For this review, take the finished solid that the model builds, in its own axes (mm). A direction names the side the tool comes from. Give positions to 0.01 mm unless a question says otherwise; leave off trailing zeros. Order: outer loops, then holes, each group sorted by start corner. A loop starts at its lowest first (then second) coordinate and runs counter-clockwise, first axis right, second up. Notation, with made-up numbers: (-6, -12) -> (13, -12) arc R20 ccw to (13, 9) -> close; hole circle Ø1 at (-2, -5.5). An arc over 180 degrees is marked (long way). Return JSON: item names as keys, results as strings. Group by question number.
1) Add section C-C (x = 0.7). Give the boundary of the cut face in (y, z).
2) Add section A-A (z = -6.5). Give the boundary of the cut face in (x, y), then the cut area to 3 significant figures.
3) For faces 4 (the face through (0.493, -11.716, 4.264)), 5 (the face through (0.49, 11.19, 0.42)), list the 3-axis set-ups (+Z, -Z, +X, -X, +Y, -Y) from which the entire face can be reached by the end or side of a thin tool; tool diameter is ignored.
4) To check wall thickness, follow line 1 along Y through (x, z) = (0.95, -6.75); line 2 along Z through (x, y) = (0.5, -10.5); line 3 along Y through (x, z) = (0.2, -12). State the ranges of each line that lie inside material, in increasing order.
5) Add section B-B (y = 0). Give the boundary of the cut face in (x, z), then the cut area to 3 significant figures.
6) The part is to be moulded in two halves that separate along Y. For faces 1 (the face through (0.493, -10.361, 6.842)), 2 (the face through (0.49, 13.19, -0.52)), 3 (the face through (0.49, -10.99, -4)), say which applies: released by +Y, released by -Y, zero draft, split by the parting line, or undercut.
7) Add section D-D (z = 7.5). Give the boundary of the cut face in (x, y).
8) Insertion check: P1, Ø8, axis at y = -8.5, z = -4.5, coming from the -X side. The pin has a flat end and moves straight along its axis. Give the tip position at first contact, or say it passes through.
from build123d import *

# Parameters (mm, degrees)
SZKIC2_R                    = 0.75
DODANIE_WYCI_GNI_CIE1_DEPTH = 1


with BuildPart() as part:
    # Szkic2 → Dodanie-wyciągnięcie1 (new body)
    with BuildSketch(Plane(origin=(0, 0, 0), x_dir=(0, 0, -1), z_dir=(1, 0, 0))):
        with BuildLine():
            Line((-4.005055878, -11.003800589), (-3.498451209, -9.611915701))
            ThreePointArc((-3.498451209, -9.611915701), (0, 11.2), (3.498451209, -9.611915701))
            Line((3.498451209, -9.611915701), (4.514665892, -12.403942594))
            ThreePointArc((4.514665892, -12.403942594), (0, 13.2), (-4.514665892, -12.403942594))
            Line((-4.514665892, -12.403942594), (-4.006558551, -11.007929147))
            Line((-4.006558551, -11.007929147), (-4.043528072, -10.989721595))
            ThreePointArc((-4.043528072, -10.989721595), (-4.024298132, -10.996777916), (-4.005055878, -11.003800589))
        make_face()
        with Locations((-6.246932231, -9.904541267)):
            Circle(SZKIC2_R, mode=Mode.SUBTRACT)
        with Locations((6.24693223, -9.904541267)):
            Circle(SZKIC2_R, mode=Mode.SUBTRACT)
    extrude(amount=DODANIE_WYCI_GNI_CIE1_DEPTH)


solid = part.part
Evaluation:
{
 "1": {"outline": "(-12.4, -4.51) arc R13.2 ccw (long way) to (-12.4, 4.51) -> (-11.01, 4.01) -> (-10.99, 4.04) arc R11.71 ccw to (-11, 4.01) -> (-9.61, 3.5) arc R10.7 cw (long way) to (-9.61, -3.5) -> close; hole circle Ø1.5 at (-9.9, -6.25); hole circle Ø1.5 at (-9.9, 6.25)"},
 "2": {"outline": "(0, -11.49) -> (1, -11.49) -> (1, -10.61) -> (0, -10.61) -> close; (0, -9.2) -> (1, -9.2) -> (1, -8) -> (0, -8) -> close; (0, 9) -> (1, 9) -> (1, 11.49) -> (0, 11.49) -> close", "area": "4.57 mm^2"},
 "3": {"face 4": "+X, -X, -Y", "face 5": "+X, -X"},
 "4": {"line 1": "-11.34 to -10.46, -9.35 to -7.8, 8.8 to 11.34", "line 2": "-8 to -6.7, -5.79 to -3.82, 3.82 to 5.79, 6.7 to 8", "line 3": "-5.5 to 5.5"},
 "5": {"outline": "(0, -13.2) -> (1, -13.2) -> (1, -10.69) -> (0, -10.69) -> close; (0, 10.69) -> (1, 10.69) -> (1, 13.2) -> (0, 13.2) -> close", "area": "5.02 mm^2"},
 "6": {"face 1": "undercut", "face 2": "split by the parting line", "face 3": "released by -Y"},
 "7": {"outline": "(0, -10.86) -> (1, -10.86) -> (1, -7.13) -> (0, -7.13) -> close; (0, 8.13) -> (1, 8.13) -> (1, 10.86) -> (0, 10.86) -> close"},
 "8": {"P1": "x = 0"}
}
